Read the model definition and answer for the solid it produces. Units are mm, in the model's axes. A direction names the side the tool comes from. Give positions to 0.01 mm unless a question says otherwise; leave off trailing zeros. Write each loop counter-clockwise with the first axis right and the second up, starting at its lowest first coordinate (ties: lowest second). Pieces come first, ordered by that corner, then holes.
```python
from build123d import *

# Parameters (mm, degrees)
SKETCH_1_R          = 4.45
EXTRUDE_1_DEPTH     = 1.9
SKETCH_2_R          = 4.45
SKETCH_2_R_2        = 3.1
CUT_EXTRUDE_2_DEPTH = 1.31
SKETCH_3_R          = 1
CUT_EXTRUDE_3_DEPTH = 3.8
CHAMFER_1_SIZE      = 0.25
CHAMFER_2_SIZE      = 2
CHAMFER_2_SIZE2     = 0.15
CHAMFER_3_SIZE      = 0.15
CHAMFER_3_SIZE2     = 2.2


with BuildPart() as part:
    # 草图1 → 拉伸1 (new, symmetric)
    with BuildSketch(Plane.XY):
        with Locations(Location((0, 0, 0), (0, 0, 180))):
            Circle(SKETCH_1_R)
    extrude(amount=EXTRUDE_1_DEPTH, both=True)

    # 草图2 → 拉伸2 (cut, symmetric)
    with BuildSketch(Plane.XY):
        with Locations(Location((0, 0, 0), (0, 0, 180))):
            Circle(SKETCH_2_R)
        Circle(SKETCH_2_R_2, mode=Mode.SUBTRACT)
    extrude(amount=CUT_EXTRUDE_2_DEPTH, both=True, mode=Mode.SUBTRACT)

    # 草图3 → 拉伸3 (cut)
    with BuildSketch(Plane.XY.offset(1.9)):
        Circle(SKETCH_3_R)
    extrude(amount=-CUT_EXTRUDE_3_DEPTH, mode=Mode.SUBTRACT)

    # 倒角1
    chamfer_1_edges = [part.edges().sort_by_distance(p)[0] for p in [
        (-1, 0, 1.9),
        (-1, 0, -1.9),
    ]]
    chamfer(chamfer_1_edges, length=CHAMFER_1_SIZE)

    # 倒角2
    chamfer_2_edges = [part.edges().sort_by_distance(p)[0] for p in [
        (4.45, 0, -1.9),
    ]]
    chamfer_2_side = [part.faces().sort_by_distance(p)[0] for p in [
        (-1.375865007, 0, -1.9),
    ]]
    chamfer(chamfer_2_edges, length=CHAMFER_2_SIZE, length2=CHAMFER_2_SIZE2, reference=chamfer_2_side[0])

    # 倒角3
    chamfer_3_edges = [part.edges().sort_by_distance(p)[0] for p in [
        (4.45, 0, 1.9),
    ]]
    chamfer_3_side = [part.faces().sort_by_distance(p)[0] for p in [
        (4.45, 0, 1.605),
    ]]
    chamfer(chamfer_3_edges, length=CHAMFER_3_SIZE, length2=CHAMFER_3_SIZE2, reference=chamfer_3_side[0])


solid = part.part
```
Item 1: Section A-A (x = 0) is taken. Write down the section's boundary in (y, z).
Result set:
outline: (-4.45, -1.75) - (-2.45, -1.9) - (-1.25, -1.9) - (-1, -1.65) - (-1, 1.65) - (-1.25, 1.9) - (-2.25, 1.9) - (-4.45, 1.75) - (-4.45, 1.31) - (-3.1, 1.31) - (-3.1, -1.31) - (-4.45, -1.31) - close; (1, -1.65) - (1.25, -1.9) - (2.45, -1.9) - (4.45, -1.75) - (4.45, -1.31) - (3.1, -1.31) - (3.1, 1.31) - (4.45, 1.31) - (4.45, 1.75) - (2.25, 1.9) - (1.25, 1.9) - (1, 1.65) - close
Item 2: Find the intervals of material crossed by line 1 along Y through (x, z) = (0, 0.8); line 2 along Z through (x, y) = (-1.75, -3.5); line 3 along Y through (x, z) = (-2, 0.5), in increasing order.
Result set:
line 1: y = -3.1 to -1, 1 to 3.1
line 2: z = -1.79 to -1.31, 1.31 to 1.79
line 3: y = -2.37 to 2.37
Item 3: Which of the six approach directions +Z, -Z, +X, -X, +Y, -Y give full straight-line access (tool end or side, diameter ignored) to faces 4 (the cylindrical face through (3.28, -3.01, 1.53)), 5 (the flat face through (-2, 3, -1.31))?
Result set:
face 4: +Z, -Z
face 5: none
Item 4: Determine the mould class of faces 1 (the flat face through (1, -1, -1.9)), 2 (the cylindrical face through (0, -1, 0)), 3 (the cylindrical face through (1.43, -2.75, -0.02)) for opening direction Y: pulls with the +Y half, pulls with the -Y half, needs draft (parallel to the pull), parting line crosses it, or undercut.
Result set:
face 1: needs draft
face 2: undercut
face 3: parting line crosses it
Item 5: Section C-C (z = 0) is taken. Write down the section's boundary in (x, y), and give its area (3 significant figures).
Result set:
outline: circle Ø6.2 at (0, 0); hole circle Ø2 at (0, 0)
area: 27.0 mm2
Item 6: Each of these flat-tipped pins is pushed along its axis until it touches: pin 1 Ø1 at (x, y) = (-3, -0.5) entering from -Z; pin 2 Ø1 at (x, z) = (-1.5, 0) entering from -Y. Where does it stop, or does it pass through?
Result set:
pin 1: stops at z = -1.89
pin 2: stops at y = -2.93
